```python
from build123d import *

# Parameters (mm, degrees)
ESBO_O1_W                 = 100
ESBO_O1_H                 = 60
RESSALTO_EXTRUS_O1_DEPTH  = 1.7
ESBO_O2_W                 = 60
ESBO_O2_H                 = 15
ESBO_O2_W_2               = 40
RESSALTO_EXTRUS_O2_DEPTH  = 13.6
RESSALTO_EXTRUS_O6_START  = 11.6
ESBO_O3_W                 = 100
ESBO_O3_H                 = 53
RESSALTO_EXTRUS_O6_DEPTH  = 1.5
ESBO_O4_W                 = 62.184169383
ESBO_O4_H                 = 2.54
ESBO_O4_W_2               = 5.08
ESBO_O4_H_2               = 42.957805244
ESBO_O4_W_3               = 56.07185462
RESSALTO_EXTRUS_O8_DEPTH  = 11.6
ESBO_O6_W                 = 21
ESBO_O6_H                 = 20
RESSALTO_EXTRUS_O9_DEPTH  = 16
ESBO_O7_W                 = 23.246964405
ESBO_O7_H                 = 12
RESSALTO_EXTRUS_O10_DEPTH = 10
ESBO_O8_R                 = 1.5
CORTE_EXTRUS_O1_DEPTH     = 10


with BuildPart() as part:
    # Esbo_o1 → Ressalto-extrus_o1 (new body)
    with BuildSketch(Plane.XY):
        Rectangle(ESBO_O1_W, ESBO_O1_H)
    extrude(amount=RESSALTO_EXTRUS_O1_DEPTH)

    # Esbo_o2 → Ressalto-extrus_o2 (add)
    with BuildSketch(Plane.XY.offset(1.7)):
        with Locations((10.7, -12.2)):
            Rectangle(ESBO_O2_W, ESBO_O2_H)
        with Locations((0.7, 10.2)):
            Rectangle(ESBO_O2_W_2, ESBO_O2_H)
    extrude(amount=RESSALTO_EXTRUS_O2_DEPTH)



with BuildPart() as body_2:
    # Esbo_o3 → Ressalto-extrus_o6 (new body)
    with BuildSketch(Plane(origin=(0, 0, 0), x_dir=(-1, 0, 0), z_dir=(0, 0, -1)).offset(RESSALTO_EXTRUS_O6_START)):
        with Locations((0, 4.4)):
            Rectangle(ESBO_O3_W, ESBO_O3_H)
    extrude(amount=RESSALTO_EXTRUS_O6_DEPTH)


with BuildPart() as part_1:
    add(part.part)

    add(body_2.part)  # Ressalto-extrus_o8 merges body 2
    # Esbo_o4 → Ressalto-extrus_o8 (add)
    with BuildSketch(Plane.XY.offset(-11.6)):
        with Locations((7.150543675, 26.719832293)):
            Rectangle(ESBO_O4_W, ESBO_O4_H)
        with Locations((45.784919315, 5.42627648)):
            Rectangle(ESBO_O4_W_2, ESBO_O4_H_2)
        with Locations((10.206701056, -18.689881399)):
            Rectangle(ESBO_O4_W_3, ESBO_O4_H)
    extrude(amount=RESSALTO_EXTRUS_O8_DEPTH)

    # Esbo_o6 → Ressalto-extrus_o9 (add)
    with BuildSketch(Plane.XY.offset(1.7)):
        with Locations((-51.5, -19)):
            Rectangle(ESBO_O6_W, ESBO_O6_H)
    extrude(amount=RESSALTO_EXTRUS_O9_DEPTH)

    # Esbo_o7 → Ressalto-extrus_o10 (add)
    with BuildSketch(Plane.XY.offset(-11.6)):
        with Locations((-45.376517798, 15.9)):
            Rectangle(ESBO_O7_W, ESBO_O7_H)
    extrude(amount=RESSALTO_EXTRUS_O10_DEPTH)

    # Esbo_o8 → Corte-extrus_o1 (cut)
    with BuildSketch(Plane(origin=(0, 0, -13.1), x_dir=(-1, 0, 0), z_dir=(0, 0, -1))):
        with Locations((34.76, 28.7)):
            Circle(ESBO_O8_R)
        with Locations((36.03, -19.56)):
            Circle(ESBO_O8_R)
        with Locations((-46.52, -19.56)):
            Circle(ESBO_O8_R)
    extrude(amount=-CORTE_EXTRUS_O1_DEPTH, mode=Mode.SUBTRACT)


solid = part_1.part
```
Work out the finished part from the listing and answer in its coordinate system (mm). A direction names the side the tool comes from. Round coordinates to 2 decimals unless told otherwise and drop trailing zeros. Write each loop counter-clockwise with the first axis right and the second up, starting at its lowest first coordinate (ties: lowest second). Pieces come first, ordered by that corner, then holes.
1) A cutting plane is placed at B-B on z = -5.5. Determine the outline of the cut face in (x, y).
2) A cutting plane is placed at C-C on x = 46.52. Determine the outline of the cut face in (y, z), and give its area (3 significant figures).
3) A cutting plane is placed at A-A on z = 11. Determine the outline of the cut face in (x, y).
4) Which of the six approach directions +Z, -Z, +X, -X, +Y, -Y give full straight-line access (tool end or side, diameter ignored) to faces 1 (the face through (0, 17.7, 8)), 2 (the face through (10, -19.7, 8)), 3 (the face through (48.325, 5, -6)), 4 (the face through (10, -19.96, -6)), 5 (the face through (-36.146, 28.125, -12.36))?
5) A cutting plane is placed at D-D on y = 15. Determine the outline of the cut face in (x, z).
6) Determine the mould class of faces 6 (the face through (-17.829, -19, -6)), 7 (the face through (10, -4.7, 8)), 8 (the face through (46, 26.905, -6)) for opening direction Y: pulls with the +Y half, pulls with the -Y half, needs draft (parallel to the pull), parting line crosses it, or undercut.
7) Consider probe 1 along Z at (x, y) = (-38.5, -14); probe 2 along Z at (x, y) = (17.5, -10.5); probe 3 along Y at (x, z) = (-2, 12.5). Determine where each line is inside the solid, lowest interval first.
8) Flat-ended cylindrical pins translate along their axes: P1, Ø10, axis at x = 10, y = -21, coming from the +Z side; P2, Ø0.8, axis at x = -15, z = -12.5, coming from the -Y side; P3, Ø10, axis at y = 17.5, z = -7.5, coming from the -X side. Find the tip coordinate at first contact, or state that the pin passes through.
Entries:
1. outline: (-57, 9.9) - (-33.75, 9.9) - (-33.75, 21.9) - (-57, 21.9) - close; (-23.94, 25.45) - (38.24, 25.45) - (38.24, 27.99) - (-23.94, 27.99) - close; (-17.83, -19.96) - (38.24, -19.96) - (38.24, -17.42) - (-17.83, -17.42) - close; (43.24, -16.05) - (48.32, -16.05) - (48.32, 26.91) - (43.24, 26.91) - close
2. outline: (-30, 0) - (-16.05, 0) - (-16.05, -11.6) - (-18.06, -11.6) - (-18.06, -13.1) - (30.9, -13.1) - (30.9, -11.6) - (26.91, -11.6) - (26.91, 0) - (30, 0) - (30, 1.7) - (-30, 1.7) - close; (-22.1, -13.1) - (-21.06, -13.1) - (-21.06, -11.6) - (-22.1, -11.6) - close
2. area: 675 mm2
3. outline: (-62, -29) - (-41, -29) - (-41, -9) - (-62, -9) - close; (-19.3, -19.7) - (40.7, -19.7) - (40.7, -4.7) - (-19.3, -4.7) - close; (-19.3, 2.7) - (20.7, 2.7) - (20.7, 17.7) - (-19.3, 17.7) - close
4. face 1: +Z, +X, -X, +Y
4. face 2: +Z, +X, -Y
4. face 3: +X, +Y, -Y
4. face 4: +X, -X, -Y
4. face 5: -Z
5. outline: (-57, -11.6) - (-50, -11.6) - (-50, -13.1) - (50, -13.1) - (50, -11.6) - (48.32, -11.6) - (48.32, 0) - (50, 0) - (50, 1.7) - (20.7, 1.7) - (20.7, 15.3) - (-19.3, 15.3) - (-19.3, 1.7) - (-50, 1.7) - (-50, 0) - (43.24, 0) - (43.24, -11.6) - (-33.75, -11.6) - (-33.75, -1.6) - (-57, -1.6) - close
6. face 6: needs draft
6. face 7: undercut
6. face 8: pulls with the +Y half
7. probe 1: z = -13.1 to -11.6, 0 to 1.7
7. probe 2: z = -13.1 to -11.6, 0 to 15.3
7. probe 3: y = -19.7 to -4.7, 2.7 to 17.7
8. P1: stops at z = 15.3
8. P2: stops at y = -22.1
8. P3: stops at x = -57
